```python
from build123d import *

# Parameters (mm, degrees)
SKETCH1_W            = 200
SKETCH1_H            = 230
BOSS_EXTRUDE1_DEPTH  = 70
SKETCH2_W            = 192
SKETCH2_H            = 222
CUT_EXTRUDE1_DEPTH   = 66
SKETCH4_W            = 196
SKETCH4_H            = 25
CUT_EXTRUDE3_DEPTH   = 10
SKETCH10_R           = 5
CUT_EXTRUDE8_DEPTH   = 167.075284133
SKETCH11_W           = 2
SKETCH11_H           = 10
BOSS_EXTRUDE2_DEPTH  = 20
SKETCH12_W           = 2
SKETCH12_H           = 5
CUT_EXTRUDE9_DEPTH   = 20
FILLET1_R            = 2.5
SKETCH13_W           = 2
SKETCH13_H           = 10
BOSS_EXTRUDE3_DEPTH  = 20
SKETCH14_W           = 2
SKETCH14_H           = 5
CUT_EXTRUDE10_DEPTH  = 20
FILLET2_R            = 2.5
SKETCH15_W           = 192
SKETCH15_H           = 66
CUT_EXTRUDE11_DEPTH  = 267.458251889
BOSS_EXTRUDE4_DEPTH  = 2
SKETCH18_R           = 7.15
CUT_EXTRUDE12_DEPTH  = 248.638849941
SKETCH19_R           = 5.05
CUT_EXTRUDE13_DEPTH  = 248.638849941
SKETCH20_R           = 5.05
CUT_EXTRUDE14_DEPTH  = 248.638849941
BOSS_EXTRUDE5_START  = 2
BOSS_EXTRUDE5_DEPTH  = 2
SKETCH21_W           = 20
SKETCH21_H           = 10
CUT_EXTRUDE15_DEPTH  = 248.638849941
SKETCH22_W           = 92
SKETCH22_H           = 40
CUT_EXTRUDE16_DEPTH  = 10
SKETCH24_R           = 5.15
CUT_EXTRUDE18_DEPTH  = 242.091269025
FILLET3_R            = 20
FILLET4_R            = 20
SKETCH25_W           = 200
SKETCH25_H           = 4.119110625
CUT_EXTRUDE19_DEPTH  = 261.384331326
SKETCH26_W           = 4
SKETCH26_H           = 65.880889375
CUT_EXTRUDE20_DEPTH  = 261.384331326
SKETCH27_W           = 4
SKETCH27_H           = 9.8
BOSS_EXTRUDE6_DEPTH  = 4.9
SKETCH28_W           = 4
SKETCH28_H           = 9.8
BOSS_EXTRUDE7_DEPTH  = 4.9
SKETCH29_R           = 12.5
SKETCH29_R_2         = 5.05
BOSS_EXTRUDE8_DEPTH  = 5
SKETCH30_R           = 8.5
SKETCH30_R_2         = 5.15
BOSS_EXTRUDE9_DEPTH  = 5
SKETCH31_R           = 10
SKETCH31_R_2         = 7.15
BOSS_EXTRUDE10_DEPTH = 4
SKETCH32_R           = 11.2
CUT_EXTRUDE21_DEPTH  = 5.5


with BuildPart() as part:
    # Sketch1 → Boss-Extrude1 (new body)
    with BuildSketch(Plane.XY):
        Rectangle(SKETCH1_W, SKETCH1_H)
    extrude(amount=BOSS_EXTRUDE1_DEPTH)

    # Sketch2 → Cut-Extrude1 (cut)
    with BuildSketch(Plane.XY.offset(70)):
        Rectangle(SKETCH2_W, SKETCH2_H)
    extrude(amount=-CUT_EXTRUDE1_DEPTH, mode=Mode.SUBTRACT)

    # Sketch4 → Cut-Extrude3 (cut)
    with BuildSketch(Plane.XZ.offset(115)):
        with Locations((0, 57.5)):
            Rectangle(SKETCH4_W, SKETCH4_H)
    extrude(amount=-CUT_EXTRUDE3_DEPTH, mode=Mode.SUBTRACT)

    # Sketch10 → Cut-Extrude8 (cut, through all)
    with BuildSketch(Plane.XY.offset(4)):
        with Locations((0, -11)):
            Circle(SKETCH10_R)
    extrude(amount=-CUT_EXTRUDE8_DEPTH, mode=Mode.SUBTRACT)

    # Sketch11 → Boss-Extrude2 (add)
    with BuildSketch(Plane.XY.offset(70)):
        with Locations((-99, -110)):
            Rectangle(SKETCH11_W, SKETCH11_H)
    extrude(amount=BOSS_EXTRUDE2_DEPTH)

    # Sketch12 → Cut-Extrude9 (cut)
    with BuildSketch(Plane.XY.offset(90)):
        with Locations((-99, -110)):
            Rectangle(SKETCH12_W, SKETCH12_H)
    extrude(amount=-CUT_EXTRUDE9_DEPTH, mode=Mode.SUBTRACT)

    # Fillet1
    fillet1_edges = [part.edges().sort_by_distance(p)[0] for p in [
        (-99, -112.5, 70),
        (-99, -107.5, 70),
    ]]
    fillet(fillet1_edges, radius=FILLET1_R - 0.0001)  # a hair under: the kernel refuses the full size

    # Sketch13 → Boss-Extrude3 (add)
    with BuildSketch(Plane.XY.offset(70)):
        with Locations((99, -110)):
            Rectangle(SKETCH13_W, SKETCH13_H)
    extrude(amount=BOSS_EXTRUDE3_DEPTH)

    # Sketch14 → Cut-Extrude10 (cut)
    with BuildSketch(Plane.XY.offset(90)):
        with Locations((99, -110)):
            Rectangle(SKETCH14_W, SKETCH14_H)
    extrude(amount=-CUT_EXTRUDE10_DEPTH, mode=Mode.SUBTRACT)

    # Fillet2
    fillet2_edges = [part.edges().sort_by_distance(p)[0] for p in [
        (99, -112.5, 70),
        (99, -107.5, 70),
    ]]
    fillet(fillet2_edges, radius=FILLET2_R - 0.0001)  # a hair under: the kernel refuses the full size

    # Sketch15 → Cut-Extrude11 (cut, through all)
    with BuildSketch(Plane(origin=(0, 115, 0), x_dir=(1, 0, 0), z_dir=(0, 1, 0))):
        with Locations((0, -37)):
            Rectangle(SKETCH15_W, SKETCH15_H)
    extrude(amount=-CUT_EXTRUDE11_DEPTH, mode=Mode.SUBTRACT)

    # Sketch16 → Boss-Extrude4 (add)
    with BuildSketch(Plane(origin=(-98, 0, 0), x_dir=(0, 0, -1), z_dir=(1, 0, 0))):
        with BuildLine():
            Line((-90, -107.5), (-72.5, -107.5))
            ThreePointArc((-72.5, -107.5), (-70, -110), (-72.5, -112.5))
            Line((-72.5, -112.5), (-90, -112.5))
            Line((-90, -112.5), (-90, -115))
            Line((-90, -115), (-45, -115))
            Line((-45, -115), (-45, -105))
            Line((-45, -105), (-90, -105))
            Line((-90, -105), (-90, -107.5))
        make_face()
    extrude(amount=BOSS_EXTRUDE4_DEPTH)

    # Sketch18 → Cut-Extrude12 (cut, through all)
    with BuildSketch(Plane(origin=(100, 0, 0), x_dir=(0, 0, -1), z_dir=(1, 0, 0))):
        with Locations((-34.45, -28.4)):
            Circle(SKETCH18_R)
    extrude(amount=-CUT_EXTRUDE12_DEPTH, mode=Mode.SUBTRACT)

    # Sketch19 → Cut-Extrude13 (cut, through all)
    with BuildSketch(Plane(origin=(100, 0, 0), x_dir=(0, 0, -1), z_dir=(1, 0, 0))):
        with Locations((-17, -95)):
            Circle(SKETCH19_R)
    extrude(amount=-CUT_EXTRUDE13_DEPTH, mode=Mode.SUBTRACT)

    # Sketch20 → Cut-Extrude14 (cut, through all)
    with BuildSketch(Plane(origin=(100, 0, 0), x_dir=(0, 0, -1), z_dir=(1, 0, 0))):
        with Locations((-17, 90)):
            Circle(SKETCH20_R)
    extrude(amount=-CUT_EXTRUDE14_DEPTH, mode=Mode.SUBTRACT)

    # Sketch17 → Boss-Extrude5 (add)
    with BuildSketch(Plane.ZY.offset(-98).offset(BOSS_EXTRUDE5_START)):
        with BuildLine():
            Line((90, -107.5), (72.5, -107.5))
            ThreePointArc((72.5, -107.5), (70, -110), (72.5, -112.5))
            Line((72.5, -112.5), (90, -112.5))
            Line((90, -112.5), (90, -115))
            Line((90, -115), (45, -115))
            Line((45, -115), (45, -105))
            Line((45, -105), (90, -105))
            Line((90, -105), (90, -107.5))
        make_face()
    extrude(amount=-BOSS_EXTRUDE5_DEPTH)

    # Sketch21 → Cut-Extrude15 (cut, through all)
    with BuildSketch(Plane(origin=(100, 0, 0), x_dir=(0, 0, -1), z_dir=(1, 0, 0))):
        with Locations((-80, -110)):
            Rectangle(SKETCH21_W, SKETCH21_H)
    extrude(amount=-CUT_EXTRUDE15_DEPTH, mode=Mode.SUBTRACT)

    # Sketch22 → Cut-Extrude16 (cut)
    with BuildSketch(Plane.XY.offset(4)):
        with Locations((0, 95)):
            Rectangle(SKETCH22_W, SKETCH22_H)
    extrude(amount=-CUT_EXTRUDE16_DEPTH, mode=Mode.SUBTRACT)

    # Sketch24 → Cut-Extrude18 (cut, through all)
    with BuildSketch(Plane(origin=(100, 0, 0), x_dir=(0, 0, -1), z_dir=(1, 0, 0))):
        with Locations((-52.45, -102)):
            Circle(SKETCH24_R)
    extrude(amount=-CUT_EXTRUDE18_DEPTH, mode=Mode.SUBTRACT)

    # Fillet3
    fillet3_edges = [part.edges().sort_by_distance(p)[0] for p in [
        (98, -115, 70),
    ]]
    fillet(fillet3_edges, radius=FILLET3_R)

    # Fillet4
    fillet4_edges = [part.edges().sort_by_distance(p)[0] for p in [
        (-98, -115, 70),
    ]]
    fillet(fillet4_edges, radius=FILLET4_R)

    # Sketch25 → Cut-Extrude19 (cut, through all)
    with BuildSketch(Plane(origin=(0, 115, 0), x_dir=(1, 0, 0), z_dir=(0, 1, 0))):
        with Locations((0, -2.059555313)):
            Rectangle(SKETCH25_W, SKETCH25_H)
    extrude(amount=-CUT_EXTRUDE19_DEPTH, mode=Mode.SUBTRACT)


with BuildPart() as cut_extrude19_piece_1:
    # of the separate pieces the step leaves, piece 1, a body of its own (cut_extrude19_pieces)
    add(part.part.solids().sort_by_distance((100, -115, 4.119110625))[0])

    # Sketch27 → Boss-Extrude6 (add)
    with BuildSketch(Plane(origin=(0, 0, 4.119110625), x_dir=(-1, 0, 0), z_dir=(0, 0, -1))):
        with Locations((-98, -86.25)):
            Rectangle(SKETCH27_W, SKETCH27_H)
    boss_extrude6 = extrude(amount=BOSS_EXTRUDE6_DEPTH)

    # Sketch28 → Boss-Extrude7 (add)
    with BuildSketch(Plane(origin=(0, 0, 4.119110625), x_dir=(-1, 0, 0), z_dir=(0, 0, -1))):
        with Locations((-98, -28.75)):
            Rectangle(SKETCH28_W, SKETCH28_H)
    boss_extrude7 = extrude(amount=BOSS_EXTRUDE7_DEPTH)

    # Mirror1: Boss-Extrude6, Boss-Extrude7 across plane
    add(boss_extrude6.mirror(Plane.ZX))
    add(boss_extrude7.mirror(Plane.ZX))

    # Sketch29 → Boss-Extrude8 (add)
    with BuildSketch(Plane.ZY.offset(-96)):
        with Locations(Location((17, 90, 0), (0, 0, 180))):
            Circle(SKETCH29_R)
        with Locations(Location((17, 90, 0), (0, 0, 180))):
            Circle(SKETCH29_R_2, mode=Mode.SUBTRACT)
    boss_extrude8 = extrude(amount=BOSS_EXTRUDE8_DEPTH)

    # Sketch30 → Boss-Extrude9 (add)
    with BuildSketch(Plane.ZY.offset(-96)):
        with Locations(Location((52.45, -102, 0), (0, 0, 180))):
            Circle(SKETCH30_R)
        with Locations(Location((52.45, -102, 0), (0, 0, 180))):
            Circle(SKETCH30_R_2, mode=Mode.SUBTRACT)
    extrude(amount=BOSS_EXTRUDE9_DEPTH)

    # Sketch31 → Boss-Extrude10 (add)
    with BuildSketch(Plane.ZY.offset(-96)):
        with Locations(Location((34.45, -28.4, 0), (0, 0, 180))):
            Circle(SKETCH31_R)
        with Locations(Location((34.45, -28.4, 0), (0, 0, 180))):
            Circle(SKETCH31_R_2, mode=Mode.SUBTRACT)
    extrude(amount=BOSS_EXTRUDE10_DEPTH)

    # Sketch32 → Cut-Extrude21 (cut)
    with BuildSketch(Plane(origin=(100, 0, 0), x_dir=(0, 0, -1), z_dir=(1, 0, 0))):
        with Locations((-17, -95)):
            Circle(SKETCH32_R)
    cut_extrude21 = extrude(amount=-CUT_EXTRUDE21_DEPTH, mode=Mode.SUBTRACT)

    # Mirror4: Boss-Extrude8 across plane
    add(boss_extrude8.mirror(Plane.ZX.offset(-2.5)))

    # Mirror5: Cut-Extrude21 across plane
    add(cut_extrude21.mirror(Plane.ZX.offset(-2.5)), mode=Mode.SUBTRACT)


with BuildPart() as cut_extrude19_piece_2:
    # of the separate pieces the step leaves, piece 2, a body of its own (cut_extrude19_pieces)
    add(part.part.solids().sort_by_distance((-100, -115, 50))[0])

    # Sketch26 → Cut-Extrude20 (cut, through all)
    with BuildSketch(Plane(origin=(0, 115, 0), x_dir=(1, 0, 0), z_dir=(0, 1, 0))):
        with Locations((-98, -37.059555313)):
            Rectangle(SKETCH26_W, SKETCH26_H)
    extrude(amount=-CUT_EXTRUDE20_DEPTH, mode=Mode.SUBTRACT)


solid = cut_extrude19_piece_1.part
```
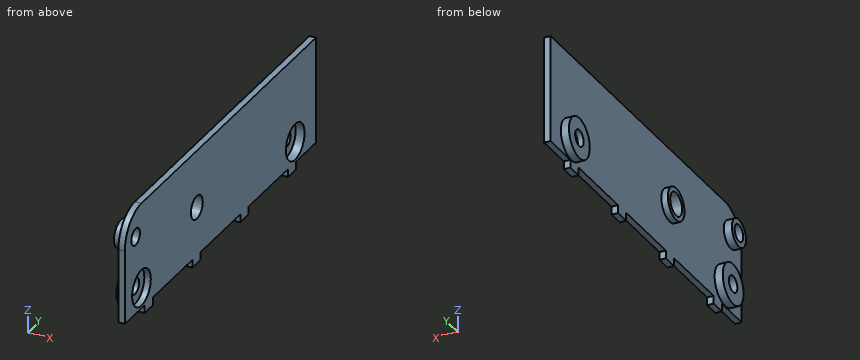
Part model, mm, in its own coordinate system. Round coordinates to 2 decimals unless told otherwise and drop trailing zeros. Loops run counter-clockwise (first coordinate to the right, second up) from the corner with the lowest first, then second, coordinate; pieces in that order, holes last. Notation, with made-up numbers: (12.5, 79.25) -> (49.5, 79.25) arc R27 ccw to (49.5, 96.25) -> close; hole circle Ø10 at (59.5, 13.25). An arc over 180 degrees is marked (long way). Use one line per item in the form item = value. Start each with the question number.
Item 1: Drop flat-ended pins along their axis: pin 1 Ø18 at (y, z) = (-98.5, 17.5) entering from +X; pin 2 Ø1.5 at (y, z) = (-42.5, 54) entering from -X; pin 3 Ø4 at (x, z) = (92.5, 44.5) entering from -Y; pin 4 Ø1.2 at (x, z) = (97.5, 2) entering from +Y. Give the stop position or say it passes through.
Item 2: Band-saw the part on C-C (x = 97.5). List the corners of the cut face in (y, z).
Item 3: Drill centre lines: line 1 along Y through (x, z) = (96.65, 17); line 2 along Y through (x, z) = (93.45, 17); line 3 along Y through (x, z) = (94.75, 34.45). Where is each one in solid material? Low to high.
Item 4: Band-saw the part on A-A (z = 34.45). List the corners of the cut face in (x, y).
Item 5: Band-saw the part on D-D (z = 17). List the corners of the cut face in (x, y), plus the area to 3 significant figures.
Item 6: Band-saw the part on B-B (y = -28.4). List the corners of the cut face in (x, z), plus the area to 3 significant figures.
Data:
q1.pin_1 = 100
q1.pin_2 = 96
q1.pin_3 = -108.07
q1.pin_4 = 91.15
q2.outline = (-115, 4.12) -> (-91.15, 4.12) -> (-91.15, -0.78) -> (-81.35, -0.78) -> (-81.35, 4.12) -> (-33.65, 4.12) -> (-33.65, -0.78) -> (-23.85, -0.78) -> (-23.85, 4.12) -> (23.85, 4.12) -> (23.85, -0.78) -> (33.65, -0.78) -> (33.65, 4.12) -> (81.35, 4.12) -> (81.35, -0.78) -> (91.15, -0.78) -> (91.15, 4.12) -> (115, 4.12) -> (115, 70) -> (-95, 70) arc R20 ccw to (-115, 50) -> close; hole circle Ø10.3 at (-102, 52.45); hole circle Ø22.4 at (-95, 17); hole circle Ø14.3 at (-28.4, 34.45); hole circle Ø22.4 at (90, 17)
q3.line_1 = -115 to -106.2, -83.8 to 78.8, 101.2 to 115
q3.line_2 = -107.5 to -100.05, -89.95 to -82.5, 77.5 to 84.95, 95.05 to 102.5
q3.line_3 = -38.4 to -35.55, -21.25 to -18.4
q4.outline = (92, -38.4) -> (96, -38.4) -> (96, -115) -> (100, -115) -> (100, -35.55) -> (92, -35.55) -> close; (92, -21.25) -> (100, -21.25) -> (100, 115) -> (96, 115) -> (96, -18.4) -> (92, -18.4) -> close
q5.outline = (91, -107.5) -> (96, -107.5) -> (96, -115) -> (100, -115) -> (100, -106.2) -> (96, -106.2) -> (96, -100.05) -> (91, -100.05) -> close; (91, -89.95) -> (96, -89.95) -> (96, -83.8) -> (100, -83.8) -> (100, 78.8) -> (94.5, 78.8) -> (94.5, 84.95) -> (91, 84.95) -> (91, 77.5) -> (96, 77.5) -> (96, -82.5) -> (91, -82.5) -> close; (91, 95.05) -> (94.5, 95.05) -> (94.5, 101.2) -> (100, 101.2) -> (100, 115) -> (96, 115) -> (96, 102.5) -> (91, 102.5) -> close
q5.area = 871 mm^2
q6.outline = (92, 24.45) -> (96, 24.45) -> (96, -0.78) -> (100, -0.78) -> (100, 27.3) -> (92, 27.3) -> close; (92, 41.6) -> (100, 41.6) -> (100, 70) -> (96, 70) -> (96, 44.45) -> (92, 44.45) -> close
q6.area = 249 mm^2
